```python
from build123d import *
from build123d.topology import SkipClean

# Parameters (mm, degrees)
BOSS_EXTRUDE1_DEPTH     = 2
BOSS_EXTRUDE2_START     = 4.5
SKETCH6_R               = 2.3
BOSS_EXTRUDE2_DEPTH     = 4.5
CUT_EXTRUDE1_DEPTH      = 33.640159313
CUT_EXTRUDE1_DEPTH_BACK = 33.640159313
SKETCH1_R               = 1.325
SKETCH7_R               = 1.75
BOSS_EXTRUDE3_DEPTH     = 3


with BuildPart() as part:
    # Sketch5 → Boss-Extrude1 (new body)
    with BuildSketch(Plane(origin=(0, 0, 0), x_dir=(1, 0, 0), z_dir=(0, 1, 0))):
        with BuildLine():
            Line((-24, 14.2), (-21.75, 12.2))
            Line((-21.75, 12.2), (21.75, 12.2))
            Line((21.75, 12.2), (24, 14.2))
            ThreePointArc((24, 14.2), (26.3, 16.5), (24, 18.8))
            Line((24, 18.8), (-24, 18.8))
            ThreePointArc((-24, 18.8), (-26.3, 16.5), (-24, 14.2))
        make_face()
    extrude(amount=BOSS_EXTRUDE1_DEPTH)

    # Sketch6 → Boss-Extrude2 (add)
    with SkipClean():  # the faces are left unmerged after this step: merging them gives an invalid solid
        with BuildSketch(Plane.XZ.offset(BOSS_EXTRUDE2_START)):
            with Locations(Location((-24, -16.5, 0), (0, 0, 270))):
                Circle(SKETCH6_R)
            with Locations(Location((24, -16.5, 0), (0, 0, 270))):
                Circle(SKETCH6_R)
        extrude(amount=-BOSS_EXTRUDE2_DEPTH)

    # Sketch1 → Cut-Extrude1 (cut, two sides: drawn at the far end of the back side and taken through both)
    with SkipClean():  # the faces are left unmerged after this step: merging them gives an invalid solid
        with BuildSketch(Plane(origin=(0, 0, 0), x_dir=(1, 0, 0), z_dir=(0, 1, 0)).offset(-CUT_EXTRUDE1_DEPTH_BACK)):
            with Locations(Location((-24, 16.5, 0), (0, 0, 270))):
                Circle(SKETCH1_R)
            with Locations(Location((24, 16.5, 0), (0, 0, 90))):
                Circle(SKETCH1_R)
            with Locations((-24, -16.5)):
                Circle(SKETCH1_R)
            with Locations((24, -16.5)):
                Circle(SKETCH1_R)
        extrude(amount=CUT_EXTRUDE1_DEPTH + CUT_EXTRUDE1_DEPTH_BACK, mode=Mode.SUBTRACT)

    # Sketch7 → Boss-Extrude3 (add)
    with SkipClean():  # the faces are left unmerged after this step: merging them gives an invalid solid
        with BuildSketch(Plane.XZ):
            with Locations(Location((-15.25, -15.25, 0), (0, 0, 90))):
                Circle(SKETCH7_R)
            with Locations(Location((15.25, -15.25, 0), (0, 0, 90))):
                Circle(SKETCH7_R)
        extrude(amount=BOSS_EXTRUDE3_DEPTH)


solid = part.part
```
Verification items for the finished model (mm, model axes). A direction names the side the tool comes from. Coordinates: 2 decimals unless noted, no trailing zeros. Order: outer loops, then holes, each group sorted by start corner. A loop starts at its lowest first (then second) coordinate and runs counter-clockwise, first axis right, second up. Notation, with made-up numbers: (38.25, 68.5) - (96.25, 68.5) arc R19 cw to (96.25, 87.5) - close; hole circle Ø4 at (50, -38). An arc over 180 degrees is marked (long way). Return JSON: item names as keys, results as strings.
(1) Access from +Z, -Z, +X, -X, +Y, -Y to the whole of each face (thin tool, end or side, straight path). Record for faces 5 (the flat face through (15, -3, -15)), 6 (the flat face through (-22.891, 0.986, -13.214)), 7 (the cylindrical face through (-16.726, -1.479, -14.309)).
Filled sheet:
{"face 5": "+Z, -Z, -Y", "face 6": "+Z, -X, +Y, -Y", "face 7": "-Y"}
(2) Mould release check, pull along X, two halves, no side actions. Record for faces 1 (the flat face through (-24, -4.5, -18)), 2 (the flat face through (0, 0, -16)), 3 (the flat face through (22.859, 0.986, -13.186)), 4 (the cylindrical face through (23.105, -1.295, -15.523)): pulls with the +X half, pulls with the -X half, needs draft (parallel to the pull), parting line crosses it, or undercut.
Filled sheet:
{"face 1": "needs draft", "face 2": "undercut", "face 3": "pulls with the +X half", "face 4": "undercut"}
(3) Section check B-B, the plane z = -16.5. Record the cut outline in (x, y) (3 decimals).
Filled sheet:
{"outline": "(-26.3, -4.5) - (-25.325, -4.5) - (-25.325, 2) - (-26.3, 2) - close; (-22.675, -4.5) - (-21.7, -4.5) - (-21.7, 0) - (-16.475, 0) - (-16.475, -3) - (-14.025, -3) - (-14.025, 0) - (14.025, 0) - (14.025, -3) - (16.475, -3) - (16.475, 0) - (21.7, 0) - (21.7, -4.5) - (22.675, -4.5) - (22.675, 2) - (-22.675, 2) - close; (25.325, -4.5) - (26.3, -4.5) - (26.3, 2) - (25.325, 2) - close"}
(4) Section check C-C, the plane y = 1.5. Record the cut outline in (x, z) (3 decimals), and give its area (3 significant figures).
Filled sheet:
{"outline": "(-24, -18.8) - (24, -18.8) arc R2.3 ccw to (24, -14.2) - (21.75, -12.2) - (-21.75, -12.2) - (-24, -14.2) arc R2.3 ccw to start; hole circle Ø2.65 at (-24, -16.5); hole circle Ø2.65 at (24, -16.5)", "area": "318 mm^2"}
(5) Section check A-A, the plane y = -2.5. Record the cut outline in (x, z) (3 decimals).
Filled sheet:
{"outline": "circle Ø4.6 at (-24, -16.5); circle Ø3.5 at (-15.25, -15.25); circle Ø3.5 at (15.25, -15.25); circle Ø4.6 at (24, -16.5); hole circle Ø2.65 at (-24, -16.5); hole circle Ø2.65 at (24, -16.5)"}
(6) Section check D-D, the plane x = -15.25. Record the cut outline in (y, z), and give its area (3 significant figures).
Filled sheet:
{"outline": "(-3, -17) - (0, -17) - (0, -18.8) - (2, -18.8) - (2, -12.2) - (0, -12.2) - (0, -13.5) - (-3, -13.5) - close", "area": "23.7 mm^2"}
(7) Thickness scan on line 1 along X through (y, z) = (0.5, -16.5) (3 decimals); line 2 along Z through (x, y) = (-24, -0.75) (3 decimals); line 3 along X through (y, z) = (0.5, -15.75). Record the ranges inside material, lowest first.
Filled sheet:
{"line 1": "x = -26.3 to -25.325, -22.675 to 22.675, 25.325 to 26.3", "line 2": "z = -18.8 to -17.825, -15.175 to -14.2", "line 3": "x = -26.17 to -25.09, -22.91 to 22.91, 25.09 to 26.17"}
(8) Go/stop test with flat-tipped pins: pin 1 (3 mm diameter, centred on x = -16, z = -14.5, fed in from -Y); pin 2 (1 mm diameter, centred on y = 0, z = -15.5, fed in from +X) (3 decimals); pin 3 (2 mm diameter, centred on x = 24, z = -16.5, fed in from +Y). Record where each tip stops, or that it passes through.
Filled sheet:
{"pin 1": "stops at y = -3", "pin 2": "stops at x = 26.245", "pin 3": "passes through"}
